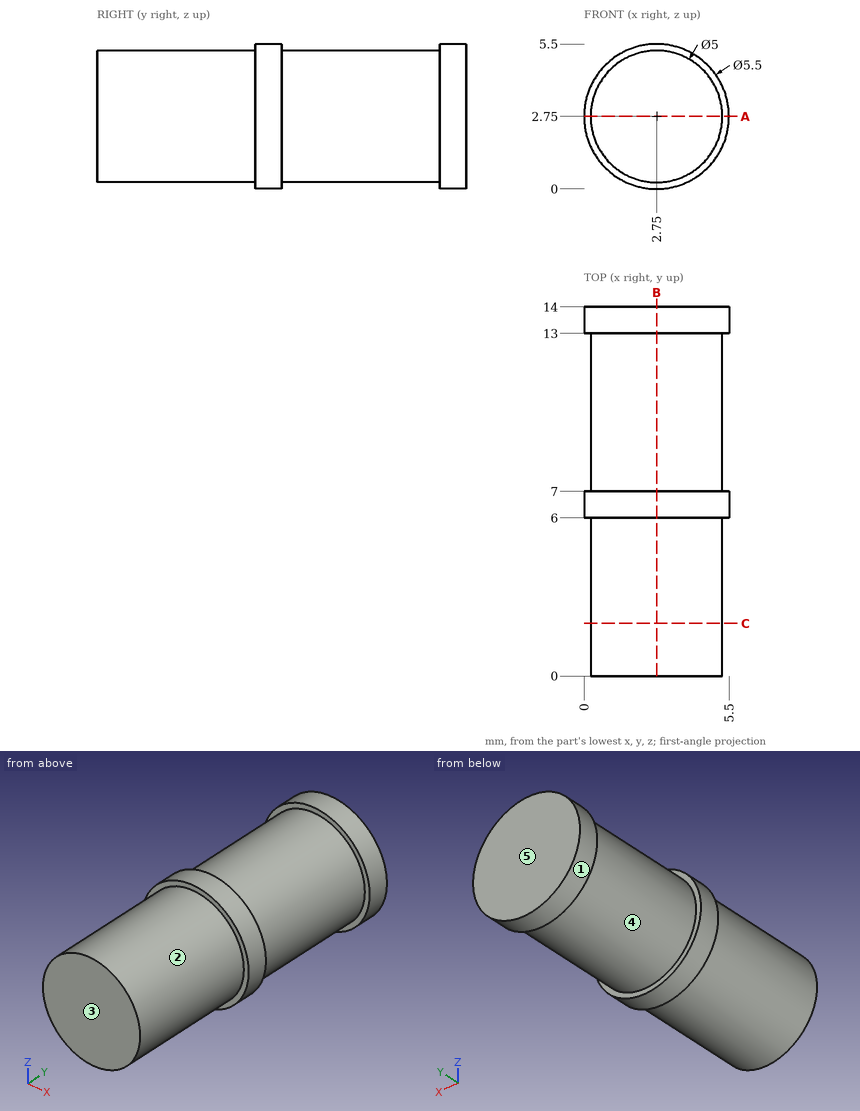
Here's the drawing with two shaded views (mm, measured from the low corner). I have some questions. A direction names the side the tool comes from. Coordinates: 2 decimals unless noted, no trailing zeros. Write each loop counter-clockwise with the first axis right and the second up, starting at its lowest first coordinate (ties: lowest second). Pieces come first, ordered by that corner, then holes. Notation, with made-up numbers: (28, 35) - (76, 35) arc R4 ccw to (76, 40) - close; hole circle Ø1 at (-40, -34.5). An arc over 180 degrees is marked (long way). Return JSON: item names as keys, results as strings.
Q1. If we section it at B-B (x = 2.75): Please give me the cut outline in (y, z).
Computed values:
{"outline": "(0, 0.25) - (6, 0.25) - (6, 0) - (7, 0) - (7, 0.25) - (13, 0.25) - (13, 0) - (14, 0) - (14, 5.5) - (13, 5.5) - (13, 5.25) - (7, 5.25) - (7, 5.5) - (6, 5.5) - (6, 5.25) - (0, 5.25) - close"}
Q2. I'm going to push flat-ended pins straight in: pin 1 Ø1.5 at (x, y) = (4.5, 11) entering from -Z; pin 2 Ø1.5 at (x, y) = (1.5, 11) entering from +Z. Where does each tip first touch, or does it pass through?
Computed values:
{"pin 1": "stops at z = 0.46", "pin 2": "stops at z = 5.2"}
Q3. If we section it at C-C (y = 2): Please give me the cut outline in (x, z).
Computed values:
{"outline": "circle Ø5 at (2.75, 2.75)"}
Q4. Please list where these lines run through material, in increasing order: L1, parallel to Z at x = 3.55, y = 5; L2, parallel to Z at x = 0.5, y = 10.75; L3, parallel to X at y = 11.75, z = 3.75. Write a range as from..to.
Computed values:
{"L1": "z = 0.38..5.12", "L2": "z = 1.66..3.84", "L3": "x = 0.46..5.04"}
Q5. On a 3-axis mill with a long thin cutter (end or side, diameter ignored), from which of +Z, -Z, +X, -X, +Y, -Y can I reach the whole of each face in a straight line? I mean the marked faces 1 and 2. Say none if no direction works.
Computed values:
{"face 1": "+Y, -Y", "face 2": "-Y"}
Q6. Thinking about a two-plate mould opening in Y: for the marked faces 3, 4 and 5, which applies, +Y half, -Y half, draft (parallel to the pull), parting line (faces both ways), or undercut?
Computed values:
{"face 3": "-Y half", "face 4": "undercut", "face 5": "+Y half"}
Q7. If we section it at A-A (z = 2.75): Please give me the cut outline in (x, y).
Computed values:
{"outline": "(0, 6) - (0.25, 6) - (0.25, 0) - (5.25, 0) - (5.25, 6) - (5.5, 6) - (5.5, 7) - (5.25, 7) - (5.25, 13) - (5.5, 13) - (5.5, 14) - (0, 14) - (0, 13) - (0.25, 13) - (0.25, 7) - (0, 7) - close"}
